Autodesk Inventor part; units mm, degrees
ref_plane "YZ Plane" through (0, 0, 0) normal (1, 0, 0) x (0, 1, 0)
ref_plane "XZ Plane" through (0, 0, 0) normal (0, 1, 0) x (-1, 0, 0)
ref_plane "XY Plane" through (0, 0, 0) normal (0, 0, 1) x (1, 0, 0)
sketch "Sketch1" plane through (0, 0, 0) normal (0, 0, 1) x (1, 0, 0)
  line L0 (-97.5, -75) -> (97.5, -75)
  line L1 (97.5, -75) -> (97.5, 75)
  line L2 (97.5, 75) -> (-97.5, 75)
  line L3 (-97.5, 75) -> (-97.5, -75)
  line L4 (-97.5, -75) -> (-32.5, -30) construction
  line L5 (97.5, -75) -> (-97.5, 75) construction
  line L6 (-97.5, -75) -> (-32.5, -75)
  line L7 (-32.5, -45) -> (-32.5, -40)
  line L8 (-42.5, 10) -> (-97.5, 10)
  line L9 (-97.5, 10) -> (-97.5, -75)
  line L10 (-97.5, -75) -> (27.5, -75)
  line L11 (27.5, -75) -> (27.5, -65)
  line L12 (17.5, -55) -> (-22.5, -55)
  line L13 (-97.5, -55) -> (-97.5, -75)
  arc A0 (-32.5, -45) -> (-22.5, -55) centre (-22.5, -45) ccw
  arc A1 (27.5, -65) -> (17.5, -55) centre (17.5, -65) ccw
  line L14 (-42.5, 10) -> (82.5, 10)
  line L15 (92.5, 0) -> (92.5, -20)
  line L16 (82.5, -30) -> (-22.5, -30)
  line L17 (-32.5, -30) -> (97.5, 75) construction
  arc A2 (-22.5, -30) -> (-32.5, -40) centre (-22.5, -40) ccw
  arc A3 (82.5, -30) -> (92.5, -20) centre (82.5, -20) ccw
  arc A4 (92.5, 0) -> (82.5, 10) centre (82.5, 0) ccw
  point P0 (0, 0)
  point P1 (-32.5, 10)
  point P2 (27.5, -55)
  point P3 (92.5, -30)
  point P4 (92.5, 10)
  dimension "d0" = 195
  dimension "d1" = 150
  dimension "d2" = 65
  dimension "d3" = 85
  dimension "d4" = 125
  dimension "d5" = 20
  dimension "d36" = 40
  dimension "d37" = 190
  dimension "d38" = 10
extrude "Extrusion1" add sketch "Sketch1" along normal blind 5 contours L11 A1 L12 A0 L7 A2 L16 A3 L15 A4 L14 L8 L3 L2 L1 L0
sketch "Sketch2" plane through (0, 0, 0) normal (0, 0, -1) x (-1, 0, 0)
  line L0 (92.5, 75) -> (97.5, 75)
  line L1 (97.5, 75) -> (97.5, 10)
  line L2 (97.5, 10) -> (92.5, 10)
  line L3 (92.5, 10) -> (92.5, 75)
  line L4 (-97.5, 75) -> (97.5, 75)
  line L5 (97.5, 10) -> (-82.5, 10)
  line L6 (97.5, 75) -> (97.5, 10)
  point P0 (0, 0)
  point P1 (42.5, 5)
  point P2 (97.5, -75)
  point P3 (-82.5, 10)
  dimension "d9" = 5
extrude "Extrusion2" add sketch "Sketch2" along normal blind 10
sketch "Sketch3" plane through (0, 0, 0) normal (0, 0, -1) x (-1, 0, 0)
  line L0 (-97.5, 75) -> (-92.5, 75)
  line L1 (-92.5, 75) -> (-92.5, -75)
  line L2 (-92.5, -75) -> (-97.5, -75)
  line L3 (-97.5, -75) -> (-97.5, 75)
  line L4 (-97.5, -70) -> (-27.5, -70)
  line L5 (-27.5, -70) -> (-27.5, -75)
  line L6 (-27.5, -75) -> (-97.5, -75)
  line L7 (-97.5, -75) -> (-97.5, -70)
  line L8 (-97.5, -75) -> (-97.5, 75)
  line L9 (-97.5, 75) -> (92.5, 75)
  line L10 (-27.5, -75) -> (-97.5, -75)
  line L11 (-27.5, -65) -> (-27.5, -75)
  point P0 (0, 0)
  point P1 (-92.5, -70)
  point P2 (97.5, -75)
  dimension "d12" = 5
  dimension "d13" = 5
extrude "Extrusion3" add sketch "Sketch3" along normal blind 20
sketch "Sketch4" plane through (97.5, -75, 5) normal (1, 0, 0) x (0, 0, -1)
  circle A0 centre (15, 30) radius 2.55
  circle A1 centre (15, 120) radius 2.55
  line L0 (0, 0) -> (0, 150)
  line L1 (25, 0) -> (0, 0)
  point P0 (5, 75)
  dimension "d16" = 5.1
  dimension "d17" = 5.1
  dimension "d18" = 15
  dimension "d19" = 30
  dimension "d20" = 90
extrude "Extrusion4" cut sketch "Sketch4" against normal blind 20
sketch "Sketch5" plane through (27.5, -75, 5) normal (0, -1, 0) x (1, 0, 0)
  circle A0 centre (35, -15) radius 2.55
  line L0 (70, -25) -> (70, 0)
  line L1 (0, 0) -> (70, 0)
  point P0 (-27.5, -5)
  point P1 (70, -12.5)
  point P2 (35, 0)
  point P3 (-125, 0)
  dimension "d23" = 5.1
  dimension "d24" = 35
  dimension "d25" = 15
extrude "Extrusion5" cut sketch "Sketch5" against normal blind 20
sketch "Sketch6" plane through (-97.5, 10, 5) normal (-1, 0, 0) x (0, 0, 1)
  circle A0 centre (-10, 45) radius 2.05
  circle A1 centre (-10, 20) radius 2.05
  line L0 (-15, 0) -> (-15, 65)
  line L1 (-15, 0) -> (0, 0)
  line L2 (0, 65) -> (-15, 65)
  point P0 (-5, -10)
  dimension "d28" = 4.1
  dimension "d29" = 4.1
  dimension "d30" = 5
  dimension "d31" = 20
  dimension "d32" = 20
extrude "Extrusion6" cut sketch "Sketch6" against normal blind 20
properties part number "tright"
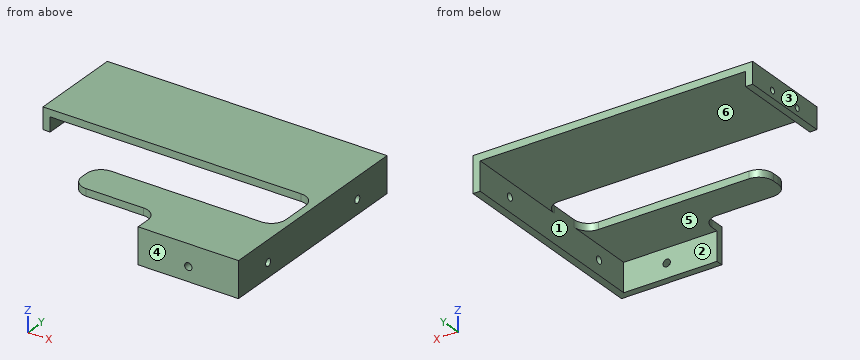
Could you check a few things on this model? Use its own coordinates, in mm. Face numbers are marked on the shaded views. A direction names the side the tool comes from. Round coordinates to 2 decimals unless told otherwise and drop trailing zeros. Loops run counter-clockwise (first coordinate to the right, second up) from the corner with the lowest first, then second, coordinate; pieces in that order, holes last. Notation, with made-up numbers: (-6, -9) - (7, -9) arc R5 cw to (7, 0) - close; hole circle Ø8 at (26.5, 35). An arc over 180 degrees is marked (long way). Answer in a Markdown table with one row per item. Add a question column.
(1) If we section it at A-A (z = -5): Please give me the cut outline in (x, y), plus the area to 3 significant figures.
(2) For the marked faces 4, 5 and 6, which set-ups out of +Z, -Z, +X, -X, +Y, -Y let a thin tool reach every point of the face, with its end or its side?
(3) I'm going to push flat-ended pins straight in: pin 1 (2 mm diameter, centred on x = 27.5, z = -8.5, fed in from +Y); pin 2 (1 mm diameter, centred on y = -42, z = -7, fed in from -X); pin 3 (8 mm diameter, centred on y = -45, z = -10, fed in from +X); pin 4 (12 mm diameter, centred on x = -42, z = 0, fed in from -Y). Where does each tip first touch, or does it pass through?
(4) If we section it at C-C (x = 62.5): Please give me the cut outline in (y, z).
(5) If we section it at D-D (x = 35.5): Please give me the cut outline in (y, z), plus the area to 3 significant figures.
(6) If we mould it in two halves opening along X, with no side actions, what happens to the marked faces 1, 2 and 3? For each: pulls with the +X half, pulls with the -X half, needs draft (parallel to the pull), parting line crosses it, or undercut.
(7) I need wall thicknesses on line 1 along Y through (x, z) = (95.25, -10); line 2 along Y through (x, z) = (-95.75, -5); line 3 along X through (y, z) = (61, -1). Which ranges of each line are inside material? Lowest first, please.
(8) If we section it at B-B (y = 30): Please give me the cut outline in (x, z).
Model answer:
| question | item | result |
|---|---|---|
| 1 | outline | (-97.5, 10) - (-92.5, 10) - (-92.5, 27.95) - (-97.5, 27.95) - close; (-97.5, 32.05) - (-92.5, 32.05) - (-92.5, 52.95) - (-97.5, 52.95) - close; (-97.5, 57.05) - (-92.5, 57.05) - (-92.5, 75) - (-97.5, 75) - close; (27.5, -75) - (97.5, -75) - (97.5, 75) - (92.5, 75) - (92.5, -70) - (27.5, -70) - close |
| 1 | area | 1,360 mm² |
| 2 | face 4 | +Z, -Z, +X, -X, -Y |
| 2 | face 5 | -Z, -X, +Y |
| 2 | face 6 | -Z, +Y |
| 3 | pin 1 | stops at y = -70 |
| 3 | pin 2 | stops at x = 92.5 |
| 3 | pin 3 | stops at x = 97.5 |
| 3 | pin 4 | stops at y = 10 |
| 4 | outline | (-75, -20) - (-70, -20) - (-70, -12.55) - (-75, -12.55) - close; (-75, -7.45) - (-70, -7.45) - (-70, 0) - (-30, 0) - (-30, 5) - (-75, 5) - close; (10, 0) - (75, 0) - (75, 5) - (10, 5) - close |
| 5 | outline | (-75, -20) - (-70, -20) - (-70, 0) - (-30, 0) - (-30, 5) - (-75, 5) - close; (10, 0) - (75, 0) - (75, 5) - (10, 5) - close |
| 5 | area | 650 mm² |
| 6 | face 1 | undercut |
| 6 | face 2 | needs draft |
| 6 | face 3 | pulls with the -X half |
| 7 | line 1 | y = -75 to -47.55, -42.45 to 42.45, 47.55 to 75 |
| 7 | line 2 | y = 10 to 27.95, 32.05 to 52.95, 57.05 to 75 |
| 7 | line 3 | x = -97.5 to -92.5, 92.5 to 97.5 |
| 8 | outline | (-97.5, -10) - (-92.5, -10) - (-92.5, -7.05) - (-97.5, -7.05) - close; (-97.5, -2.95) - (-92.5, -2.95) - (-92.5, 0) - (92.5, 0) - (92.5, -20) - (97.5, -20) - (97.5, 5) - (-97.5, 5) - close |
